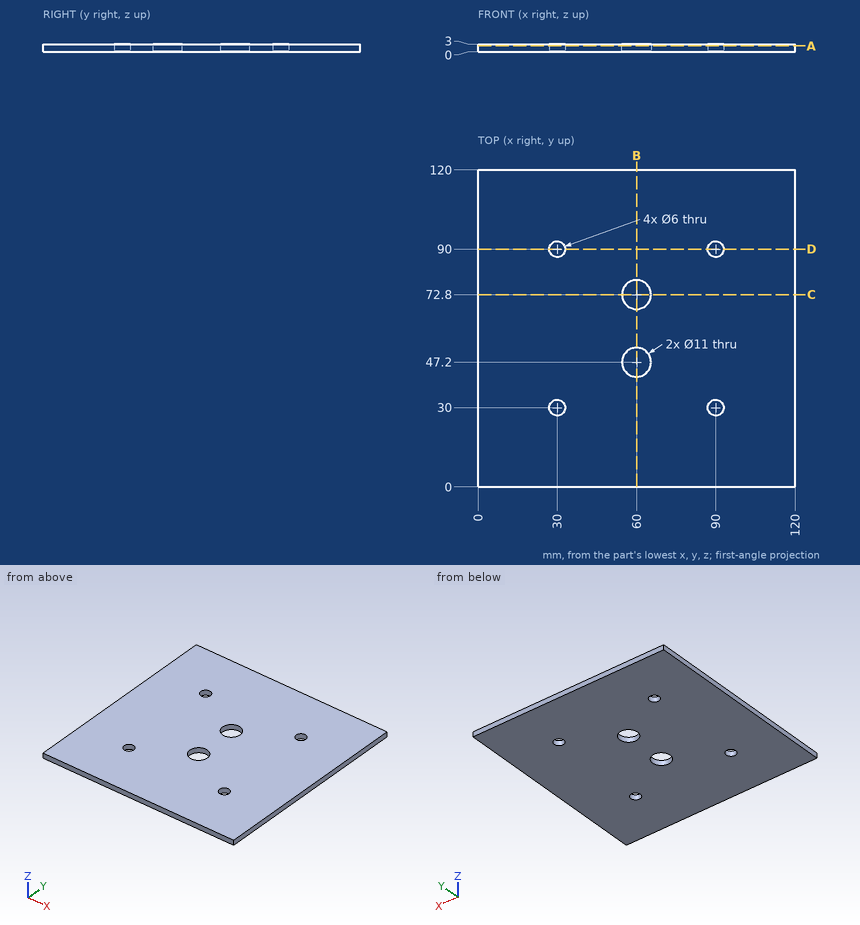
Job drawing, mm, ordinate dimensions from the low corner. One solid piece. Coordinates: 2 decimals unless noted, no trailing zeros. Order: outer loops, then holes, each group sorted by start corner. A loop starts at its lowest first (then second) coordinate and runs counter-clockwise, first axis right, second up. Notation, with made-up numbers: (33, 71.25) - (38, 71.25) arc R17 ccw to (38, 75.25) - close; hole circle Ø8 at (28.25, 15). An arc over 180 degrees is marked (long way). Write each question's results on one line, items separated by ' | '. Start each with the question number.
Item 1: Band-saw the part on B-B on x = 60. Write the cut outline in (y, z).
Item 2: Band-saw the part on A-A on z = 2.3. Write the cut outline in (x, y).
Item 3: Band-saw the part on D-D on y = 90. Write the cut outline in (x, z).
Item 4: Wall check: probe 1 along Y at (x, z) = (30, 1.25); probe 2 along Y at (x, z) = (60, 1.85); probe 3 along X at (y, z) = (29, 2.2). Give the ranges that are in metal, low to high. Write a range as [from, to].
Item 5: Band-saw the part on C-C on y = 72.8. Write the cut outline in (x, z).
Numbers:
1) outline: (0, 0) - (41.7, 0) - (41.7, 3) - (0, 3) - close; (52.7, 0) - (67.3, 0) - (67.3, 3) - (52.7, 3) - close; (78.3, 0) - (120, 0) - (120, 3) - (78.3, 3) - close
2) outline: (0, 0) - (120, 0) - (120, 120) - (0, 120) - close; hole circle Ø6 at (30, 30); hole circle Ø6 at (30, 90); hole circle Ø11 at (60, 47.2); hole circle Ø11 at (60, 72.8); hole circle Ø6 at (90, 30); hole circle Ø6 at (90, 90)
3) outline: (0, 0) - (27, 0) - (27, 3) - (0, 3) - close; (33, 0) - (87, 0) - (87, 3) - (33, 3) - close; (93, 0) - (120, 0) - (120, 3) - (93, 3) - close
4) probe 1: [0, 27], [33, 87], [93, 120] | probe 2: [0, 41.7], [52.7, 67.3], [78.3, 120] | probe 3: [0, 27.17], [32.83, 87.17], [92.83, 120]
5) outline: (0, 0) - (54.5, 0) - (54.5, 3) - (0, 3) - close; (65.5, 0) - (120, 0) - (120, 3) - (65.5, 3) - close
